The model under review builds one solid part; all positions refer to its coordinate system, in mm. A direction names the side the tool comes from. Give positions to 0.01 mm unless a question says otherwise; leave off trailing zeros. Write each loop counter-clockwise with the first axis right and the second up, starting at its lowest first coordinate (ties: lowest second). Pieces come first, ordered by that corner, then holes. Notation, with made-up numbers: M -17.75,49.25 L 11.25,49.25 A13 cw 11.25,54.25 Z; hole C 32.25,-38 d1. An arc over 180 degrees is marked long. Write item = value, one per line. Start each with the question number.
```python
from build123d import *

# Parameters (mm, degrees)
BOSS_EXTRUDE1_DEPTH                    = 2
BOSS_EXTRUDE2_START                    = -2.54
SKETCH5_R                              = 5.00000016
BOSS_EXTRUDE2_DEPTH                    = 2.54
F_18_0_1695_DIAMETER_HOLE1_D           = 4.3053
F_18_0_1695_DIAMETER_HOLE1_DEPTH       = 4.572
F_18_0_1695_DIAMETER_HOLE1_CSINK_D     = 5.08
F_18_0_1695_DIAMETER_HOLE1_CSINK_ANGLE = 90
F_18_0_1695_DIAMETER_HOLE1_TIP         = 1.293442612
SKETCH3_R                              = 4.5
SKETCH3_R_2                            = 0.97241532
SKETCH3_W                              = 27.07
SKETCH3_H                              = 15.132
CUT_EXTRUDE1_DEPTH                     = 64.648399546
CHAMFER1_SIZE                          = 0.508


with BuildPart() as part:
    # Sketch1 → Boss-Extrude1 (new body)
    with BuildSketch(Plane.XY):
        with BuildLine():
            Line((-52.07, 5.00000016), (-57.07000016, 5.00000016))
            ThreePointArc((-57.07000016, 5.00000016), (-62.07000032, 0), (-57.07000016, -5.00000016))
            Line((-57.07000016, -5.00000016), (-52.07, -5.00000016))
            Line((-52.07, -5.00000016), (-52.07, -13.335))
            Line((-52.07, -13.335), (52.07, -13.335))
            Line((52.07, -13.335), (52.07, -5.00000016))
            Line((52.07, -5.00000016), (57.07000016, -5.00000016))
            ThreePointArc((57.07000016, -5.00000016), (62.07000032, 0), (57.07000016, 5.00000016))
            Line((57.07000016, 5.00000016), (52.07, 5.00000016))
            Line((52.07, 5.00000016), (52.07, 13.335))
            Line((52.07, 13.335), (-52.07, 13.335))
            Line((-52.07, 13.335), (-52.07, 5.00000016))
        make_face()
    extrude(amount=BOSS_EXTRUDE1_DEPTH)

    # Sketch5 → Boss-Extrude2 (add)
    with BuildSketch(Plane.XY.offset(BOSS_EXTRUDE2_START)):
        with Locations(Location((-57.07000016, 0, 0), (0, 0, 90))):
            Circle(SKETCH5_R)
        with Locations(Location((57.07000016, 0, 0), (0, 0, 270))):
            Circle(SKETCH5_R)
    extrude(amount=BOSS_EXTRUDE2_DEPTH)

    # #18 (0.1695) Diameter Hole1
    with Locations(Plane(origin=(0, 0, -2.54), x_dir=(-1, 0, 0), z_dir=(0, 0, -1))):
        with Locations((57.07000016, 0), (-57.07000016, 0)):
            CounterSinkHole(F_18_0_1695_DIAMETER_HOLE1_D / 2, F_18_0_1695_DIAMETER_HOLE1_CSINK_D / 2, depth=F_18_0_1695_DIAMETER_HOLE1_DEPTH, counter_sink_angle=F_18_0_1695_DIAMETER_HOLE1_CSINK_ANGLE)
            with Locations((0, 0, -(F_18_0_1695_DIAMETER_HOLE1_DEPTH + F_18_0_1695_DIAMETER_HOLE1_TIP / 2))):  # 118° drill point
                Cone(0, F_18_0_1695_DIAMETER_HOLE1_D / 2, F_18_0_1695_DIAMETER_HOLE1_TIP, mode=Mode.SUBTRACT)

    # Sketch3 → Cut-Extrude1 (cut, through all)
    with BuildSketch(Plane.XY.offset(2)):
        with Locations((31.240005277, 0)):
            Circle(SKETCH3_R)
        with Locations((25.010807092, 0)):
            Circle(SKETCH3_R_2)
        with Locations((-4.079994723, 2.413)):
            Rectangle(SKETCH3_W, SKETCH3_H)
        with Locations((-32.269994731, 2.413)):
            Rectangle(SKETCH3_W, SKETCH3_H)
    extrude(amount=-CUT_EXTRUDE1_DEPTH, mode=Mode.SUBTRACT)

    # Chamfer1
    chamfer1_edges = [part.edges().sort_by_distance(p)[0] for p in [
        (-18.734994731, 2.413, 2),
        (-32.269994731, 9.979, 2),
        (-45.804994731, 2.413, 2),
        (-32.269994731, -5.153, 2),
        (-17.614994723, 2.413, 2),
        (-4.079994723, -5.153, 2),
        (9.455005277, 2.413, 2),
        (-4.079994723, 9.979, 2),
    ]]
    chamfer(chamfer1_edges, length=CHAMFER1_SIZE)


solid = part.part
```
Item 1: To check wall thickness, follow probe 1 along Y at (x, z) = (-15, 0.75) (3 decimals); probe 2 along X at (y, z) = (4, 0.65) (3 decimals); probe 3 along Z at (x, y) = (-26, -7.25). State the ranges of each line that lie inside material, in increasing order. Write a range as [from, to].
Item 2: The part is to be moulded in two halves that separate along Y. For faces 6 (the flat face through (-55, 5, 1)), 7 (the cylindrical face through (59.123, 0.647, -0.047)), 8 (the flat face through (-55, -5, 1)), 9 (the flat face through (52.07, -9, 1)), say which applies: released by +Y, released by -Y, zero draft, split by the parting line, or undercut.
Item 3: We need section D-D, the plane y = -10.5. Write out the cut boundary in (x, z), and give its area (3 significant figures).
Item 4: We need section A-A, the plane y = 6.25. Write out the cut boundary in (x, z) (3 decimals), and give its area (3 significant figures).
Item 5: For faces 1 (the flat face through (52.07, 9, 1)), 2 (the cylindrical face through (62.027, 0.651, -0.806)), 3 (the flat face through (-55, 2, -2.54)), 4 (the cylindrical face through (-59.22, 0.09, -0.05)), 5 (the flat face through (-52.07, 9, 1)), list the 3-axis set-ups (+Z, -Z, +X, -X, +Y, -Y) from which the entire face can be reached by the end or side of a thin tool; tool diameter is ignored.
Item 6: Clearance check with flat-ended pins moving along their axes: P1, Ø2, axis at y = 8.5, z = 0.5, coming from the +X side; P2, Ø1, axis at x = 53.5, z = 1, coming from the +Y side; P3, Ø0.7, axis at y = 2, z = 1, coming from the +X side. State where each tip first meets the part, or that it passes through.
Item 7: We need section C-C, the plane x = 12. Write out the cut boundary in (y, z) (3 decimals), and give its area (3 significant figures).
Item 8: We need section B-B, the plane z = -1.3. Write out the cut boundary in (x, y), and give its area (3 significant figures).
Worked out:
q1.probe_1 = [-13.335, -5.153], [9.979, 13.335]
q1.probe_2 = [-60.07, -45.805], [-18.735, -17.615], [9.455, 29.178], [33.302, 60.07]
q1.probe_3 = [0, 2]
q2.face_6 = released by +Y
q2.face_7 = undercut
q2.face_8 = released by -Y
q2.face_9 = zero draft
q3.outline = M -52.07,0 L 52.07,0 L 52.07,2 L -52.07,2 Z
q3.area = 208 mm²
q4.outline = M -52.07,0 L -45.805,0 L -45.805,1.492 L -46.313,2 L -52.07,2 Z; M -18.735,0 L -17.615,0 L -17.615,1.492 L -18.123,2 L -18.227,2 L -18.735,1.492 Z; M 9.455,0 L 52.07,0 L 52.07,2 L 9.963,2 L 9.455,1.492 Z
q4.area = 99.5 mm²
q5.face_1 = +Z, -Z, +X, +Y
q5.face_2 = -Z
q5.face_3 = -Z, +X, -X, +Y, -Y
q5.face_4 = +Z, -Z
q5.face_5 = +Z, -Z, -X, +Y
q6.P1 = 52.07
q6.P2 = 5
q6.P3 = 61.79
q7.outline = M -13.335,0 L 13.335,0 L 13.335,2 L -13.335,2 Z
q7.area = 53.3 mm²
q8.outline = C -57.07,0 d10; C 57.07,0 d10; hole C -57.07,0 d4.31; hole C 57.07,0 d4.31
q8.area = 128 mm²
